Can you work these out from the model? Positions are in its coordinate system, mm. Give positions to 0.01 mm unless a question says otherwise; leave off trailing zeros. Order: outer loops, then holes, each group sorted by start corner. A loop starts at its lowest first (then second) coordinate and runs counter-clockwise, first axis right, second up. Notation, with made-up numbers: M 4.25,71 L 16.25,71 A18 ccw 16.25,82 Z; hole C 28,-13.75 d2. An arc over 180 degrees is marked long. Use one line per item in the form item = value. Start each with the question number.
1. I want a section at A-A, the plane z = 16. List the corners of the cut face in (x, y) for me, and give its area (3 significant figures).
2. Will these pins go through, and if not, where does the flat tip stop? P1, Ø1, axis at x = 5.5, y = 5, coming from the +Z side; P2, Ø6, axis at x = 8, z = 4.5, coming from the +Y side (3 decimals); P3, Ø2, axis at x = 7.5, y = 13, coming from the -Z side.
3. I want a section at D-D, the plane y = 26. List the corners of the cut face in (x, z) for me, and give its area (3 significant figures).
4. I need wall thicknesses on L1, parallel to Y at x = 11.5, z = 24; L2, parallel to Y at x = 10.75, z = 36; L3, parallel to Y at x = 2.75, z = 8. Which ranges of each line are inside material? Lowest first, please.
5. I want a section at B-B, the plane y = 6. List the corners of the cut face in (x, z) for me, and give its area (3 significant figures).
6. We'd pull the mould along Z, two halves only. Please class faces 1 (the face through (7.6, 3.78, 25.59)), 2 (the face through (7.6, 3.78, 17.59)), 3 (the face through (7, 0, 20)), 4 (the face through (7.395, 17.745, 10.14)): +Z half, -Z half, draft (parallel to the pull), parting line (faces both ways), or undercut.
7. I want a section at C-C, the plane x = 5.75. List the corners of the cut face in (y, z) for me, and give its area (3 significant figures).
Autodesk Fusion 360 part; units mm, degrees
sketch "Sketch1" plane through (0, 0, 0) normal (1, 0, 0) x (0, 0, -1)
  line L0 (0, 0) -> (-40, 0)
  line L1 (-20, 0) -> (-20, 35)
  line L2 (-20, 35) -> (-40, 0)
  line L3 (-20, 35) -> (0, 0)
  dimension "d1" = 40
  dimension "d2" = 40.3113
extrude "Extrude1" add sketch "Sketch1" along normal blind 5
extrude "Extrude2" add 1 faces at (5, 11.6667, 20) along direction (1, 0, 0) blind 10
sketch "Sketch2" plane through (15, 0, 0) normal (1, 0, 0) x (0, 0, -1)
  line L0 (-20, 35) -> (-40, 0)
  line L1 (-40, 0) -> (0, 0)
  line L2 (0, 0) -> (-20, 35)
  circle A0 centre (-24, 4.9922) radius 2
  circle A1 centre (-16, 4.9922) radius 2
  line L3 (-20, 35) -> (-20, 0)
  dimension "d7" = 4
  dimension "d8" = 4
  dimension "d9" = 4
  dimension "d10" = 4
extrude "Extrude3" cut sketch "Sketch2" against normal blind 31 contours A0 | A1
Check result:
q1.outline = M 0,0 L 15,0 L 15,2.99 L 0,2.99 Z; M 0,6.99 L 15,6.99 L 15,28 L 0,28 Z
q1.area = 360 mm2
q2.P1 = 37.43
q2.P2 = 13.125
q2.P3 = 6.86
q3.outline = M 0,14.86 L 15,14.86 L 15,25.14 L 0,25.14 Z
q3.area = 154 mm2
q4.L1 = 0 to 2.99, 6.99 to 28
q4.L2 = 0 to 7
q4.L3 = 0 to 14
q5.outline = M 0,3.43 L 15,3.43 L 15,14.27 L 0,14.27 Z; M 0,17.73 L 15,17.73 L 15,22.27 L 0,22.27 Z; M 0,25.73 L 15,25.73 L 15,36.57 L 0,36.57 Z
q5.area = 393 mm2
q6.face_1 = undercut
q6.face_2 = undercut
q6.face_3 = draft
q6.face_4 = -Z half
q7.outline = M 0,0 L 35,20 L 0,40 Z; hole C 4.99,16 d4; hole C 4.99,24 d4
q7.area = 675 mm2
